Read the model definition and answer for the solid it produces. Units are mm, in the model's axes. Round coordinates to 2 decimals unless told otherwise and drop trailing zeros. Loops run counter-clockwise (first coordinate to the right, second up) from the corner with the lowest first, then second, coordinate; pieces in that order, holes last. Notation, with made-up numbers: (69, 69) - (81, 69) arc R11 ccw to (81, 78) - close; hole circle Ø1 at (-17, 19.25). An arc over 180 degrees is marked (long way). Use one line per item in the form item = value. Start each with the question number.
```python
from build123d import *

# Parameters (mm, degrees)
SKETCH1_W           = 40
SKETCH1_H           = 10
BOSS_EXTRUDE1_DEPTH = 140
FILLET4_RADIUS      = 20
FILLET4_LENGTH      = 10
SKETCH2_R           = 2.65
CUT_EXTRUDE1_DEPTH  = 10
FILLET5_R           = 5


with BuildPart() as part:
    # Sketch1 → Boss-Extrude1 (new body)
    with BuildSketch(Plane(origin=(0, 0, 0), x_dir=(1, 0, 0), z_dir=(0, 1, 0))):
        with Locations((-15.258586642, -11.19989116)):
            Rectangle(SKETCH1_W, SKETCH1_H)
    extrude(amount=BOSS_EXTRUDE1_DEPTH)

    # Fillet4: full round fillet: the end face becomes a half cylinder, R = half its width
    fillet4_face = Plane((-15.258586642, 140, 11.19989116), x_dir=(0, 0, -1), z_dir=(0, 1, 0))  # on the end face: x along it, z out of the body
    fillet4_slab = fillet4_face.offset(-FILLET4_RADIUS / 2) * Box(FILLET4_LENGTH, 2 * FILLET4_RADIUS, FILLET4_RADIUS, mode=Mode.PRIVATE)  # the body's end, R deep
    fillet4_round = Plane((-15.258586642, 120, 11.19989116), x_dir=(0, 1, 0), z_dir=(0, 0, -1)) * Cylinder(FILLET4_RADIUS, FILLET4_LENGTH, mode=Mode.PRIVATE)  # its axis R under the face
    add(fillet4_slab - fillet4_round, mode=Mode.SUBTRACT)

    # Sketch2 → Cut-Extrude1 (cut)
    with BuildSketch(Plane(origin=(0, 0, 6.19989116), x_dir=(-1, 0, 0), z_dir=(0, 0, -1))):
        with Locations((5.358586642, 10)):
            Circle(SKETCH2_R)
        with Locations((25.358586642, 10)):
            Circle(SKETCH2_R)
        with Locations((25.358586642, 30)):
            Circle(SKETCH2_R)
        with Locations((5.358586642, 30)):
            Circle(SKETCH2_R)
    extrude(amount=-CUT_EXTRUDE1_DEPTH, mode=Mode.SUBTRACT)

    # Fillet5
    fillet5_edges = [part.edges().sort_by_distance(p)[0] for p in [
        (-15.258586642, 0, 16.19989116),
        (-15.258586642, 0, 6.19989116),
    ]]
    fillet(fillet5_edges, radius=FILLET5_R - 0.0001)  # a hair under: the kernel refuses the full size


solid = part.part
```
1) Straight lines are drawn through the part: line 1 (Y direction, x = -26.5, z = 14.25); line 2 (Y direction, x = -27, z = 15.25); line 3 (Y direction, x = -15.5, z = 14.75). For each, find the intervals that lie inside material, in ascending order. Write a range as from..to.
2) A cutting plane is placed at B-B on z = 10. Write down the section's boundary in (x, y), plus the area to 3 significant figures.
3) A cutting plane is placed at A-A on y = 10. Write down the section's boundary in (x, z), plus the area to 3 significant figures.
4) Flat-ended cylindrical pins translate along their axes: pin 1 (7 mm diameter, centred on x = -25.36, y = 10, fed in from -Z); pin 2 (4 mm diameter, centred on x = -28.5, z = 14.5, fed in from +Y); pin 3 (6 mm diameter, centred on x = -2.5, z = 13, fed in from +Y); pin 4 (1.5 mm diameter, centred on x = -29.5, z = 8, fed in from +Y). Find the tip coordinate at first contact, or state that the pin passes through.
5) Determine the mould class of faces 1 (the cylindrical face through (-23.256, 8.388, 11.13)), 2 (the cylindrical face through (-15.698, 139.995, 11.13)), 3 (the flat face through (4.741, 59, 11)) for opening direction Y: +Y half, -Y half, draft (parallel to the pull), parting line (faces both ways), or undercut.
Checks:
q1.line_1 = 1.04..7.61, 12.39..27.61, 32.39..136.54
q1.line_2 = 2.07..7.92, 12.08..27.92, 32.08..136.19
q1.line_3 = 1.48..140
q2.outline = (-35.26, 0.15) - (4.74, 0.15) - (4.74, 120) arc R20 ccw to (-35.26, 120) - close; hole circle Ø5.3 at (-25.36, 10); hole circle Ø5.3 at (-25.36, 30); hole circle Ø5.3 at (-5.36, 10); hole circle Ø5.3 at (-5.36, 30)
q2.area = 5,330 mm²
q3.outline = (-35.26, 6.2) - (-28.01, 6.2) - (-28.01, 16.2) - (-35.26, 16.2) - close; (-22.71, 6.2) - (-8.01, 6.2) - (-8.01, 16.2) - (-22.71, 16.2) - close; (-2.71, 6.2) - (4.74, 6.2) - (4.74, 16.2) - (-2.71, 16.2) - close
q3.area = 294 mm²
q4.pin_1 = 6.2
q4.pin_2 = 136.54
q4.pin_3 = 137.46
q4.pin_4 = 134.76
q5.face_1 = undercut
q5.face_2 = +Y half
q5.face_3 = draft
